The figure shows three views and two pictorial views of one solid part (mm, origin at its lowest corner). Answer the questions. Coordinates: 2 decimals unless noted, no trailing zeros. Order: outer loops, then holes, each group sorted by start corner. A loop starts at its lowest first (then second) coordinate and runs counter-clockwise, first axis right, second up. Notation, with made-up numbers: (31.25, 52.5) -> (74.25, 52.5) arc R30 ccw to (74.25, 74.5) -> close; hole circle Ø10 at (-32.5, 20). An arc over 180 degrees is marked (long way). Return JSON: item names as keys, results as strings.
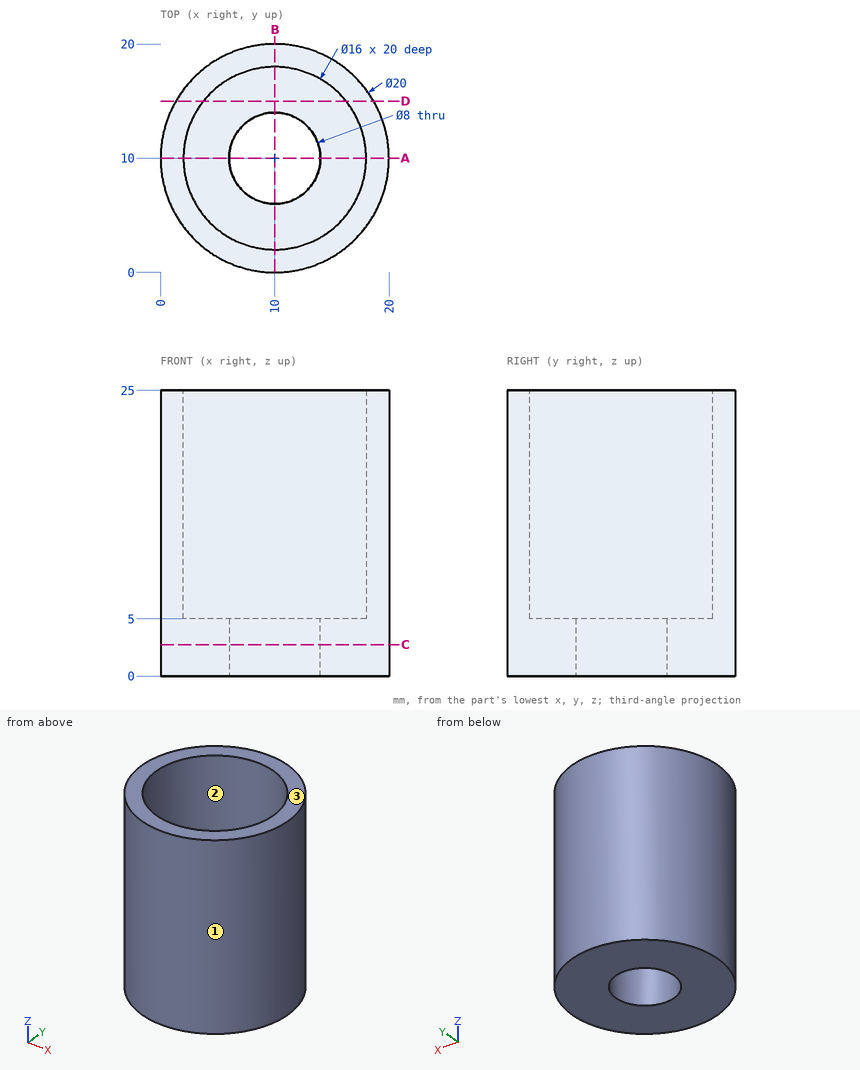
Item 1: Determine the mould class of the marked faces 1, 2 and 3 for opening direction Y: pulls with the +Y half, pulls with the -Y half, needs draft (parallel to the pull), parting line crosses it, or undercut.
Answer list:
{"face 1": "parting line crosses it", "face 2": "undercut", "face 3": "needs draft"}
Item 2: Flat-ended cylindrical pins translate along their axes: pin 1 (2 mm diameter, centred on x = 15.5, z = 18, fed in from -Y); pin 2 (1.5 mm diameter, centred on y = 7, z = 9, fed in from +X); pin 3 (3 mm diameter, centred on x = 15, z = 22, fed in from +Y). Find the tip coordinate at first contact, or state that the pin passes through.
Answer list:
{"pin 1": "y = 1.07", "pin 2": "x = 19.74", "pin 3": "y = 19.37"}
Item 3: The part is cut by section C-C on z = 2.75. Determine the outline of the cut face in (x, y), plus the area to 3 significant figures.
Answer list:
{"outline": "circle Ø20 at (10, 10); hole circle Ø8 at (10, 10)", "area": "264 mm2"}
Item 4: The part is cut by section A-A on y = 10. Determine the outline of the cut face in (x, z), plus the area to 3 significant figures.
Answer list:
{"outline": "(0, 0) -> (6, 0) -> (6, 5) -> (2, 5) -> (2, 25) -> (0, 25) -> close; (14, 0) -> (20, 0) -> (20, 25) -> (18, 25) -> (18, 5) -> (14, 5) -> close", "area": "140 mm2"}
Item 5: Find the intervals of material crossed by probe 1 along Y at (x, z) = (10, 2.55); probe 2 along Y at (x, z) = (10, 17.75); probe 3 along Z at (x, y) = (2.75, 11), in increasing order.
Answer list:
{"probe 1": "0 to 6, 14 to 20", "probe 2": "0 to 2, 18 to 20", "probe 3": "0 to 5"}
Item 6: The part is cut by section D-D on y = 15. Determine the outline of the cut face in (x, z) (3 decimals), plus the area to 3 significant figures.
Answer list:
{"outline": "(1.34, 0) -> (18.66, 0) -> (18.66, 25) -> (16.245, 25) -> (16.245, 5) -> (3.755, 5) -> (3.755, 25) -> (1.34, 25) -> close", "area": "183 mm2"}
